Can you work these out from the drawing? Everything is in mm from the part's minimum corner. Give positions to 0.01 mm unless a question says otherwise; leave off trailing zeros. Order: outer loops, then holes, each group sorted by start corner. A loop starts at its lowest first (then second) coordinate and runs counter-clockwise, first axis right, second up. Notation, with made-up numbers: M -32.75,-10 L 4.25,-10 A25 ccw 4.25,9 Z; hole C 39,50 d5. An arc over 180 degrees is marked long. Answer as a JSON object with one key per item and string values.
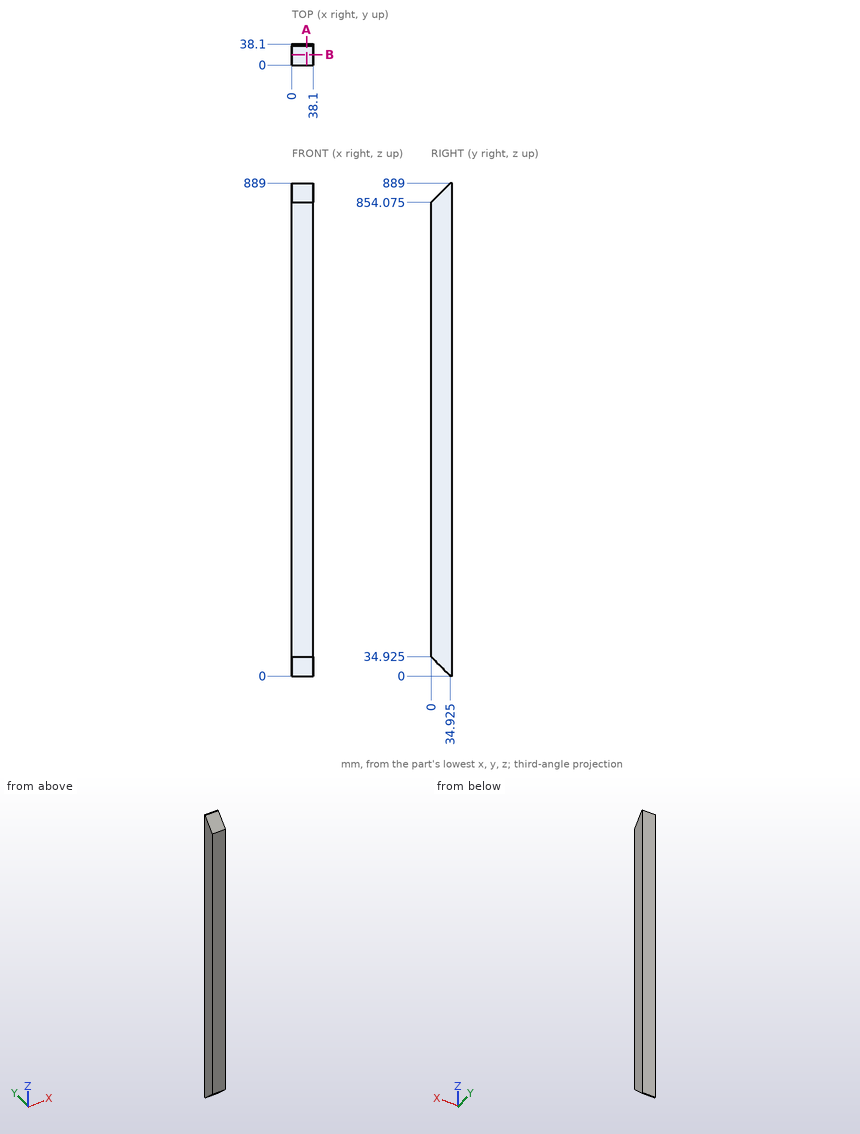
1) I want a section at A-A on x = 26.5. Write out the boundary of the cut face in (y, z) (3 decimals), and give its area (3 significant figures).
Results found:
{"outline": "M 0,34.925 L 34.925,0 L 38.1,0 L 38.1,889 L 34.925,889 L 0,854.075 Z", "area": "32,700 mm²"}
2) I'm going to push flat-ended pins straight in: pin 1 Ø12 at (x, y) = (12, 28) entering from -Z (3 decimals); pin 2 Ø3 at (x, y) = (14.5, 26) entering from +Z (3 decimals); pin 3 Ø2 at (x, y) = (34, 21) entering from -Z (3 decimals). Where does each tip first touch, or does it pass through?
Results found:
{"pin 1": "stops at z = 0.925", "pin 2": "stops at z = 881.575", "pin 3": "stops at z = 12.925"}
3) I need wall thicknesses on L1, parallel to Z at x = 28.5, y = 16 (3 decimals); L2, parallel to Z at x = 19, y = 9 (3 decimals). Which ranges of each line are inside material? Lowest first, please.
Results found:
{"L1": "z = 18.925 to 870.075", "L2": "z = 25.925 to 863.075"}
4) I want a section at B-B on y = 19. Write out the boundary of the cut face in (x, z) (3 decimals), and give its area (3 significant figures).
Results found:
{"outline": "M 0,15.925 L 38.1,15.925 L 38.1,873.075 L 0,873.075 Z", "area": "32,700 mm²"}
